Read the model definition and answer for the solid it produces. Units are mm, in the model's axes. A direction names the side the tool comes from. Round coordinates to 2 decimals unless told otherwise and drop trailing zeros. Order: outer loops, then holes, each group sorted by start corner. A loop starts at its lowest first (then second) coordinate and runs counter-clockwise, first axis right, second up. Notation, with made-up numbers: (33.25, 37.25) - (50.25, 37.25) arc R27 cw to (50.25, 75.25) - close; hole circle Ø8 at (-16, 22). An arc over 180 degrees is marked (long way). One line per question, with ' | ' between items. Start each with the question number.
1) Straight lines are drawn through the part: line 1 (X direction, y = 0, z = -6); line 2 (X direction, y = 0, z = -1.3); line 3 (Z direction, x = -1.75, y = 4.5). For each, find the intervals that lie inside material, in ascending order. Write a range as from..to.
2) The mould has two halves that part along Y. Classify faces 4 (the cylindrical face through (-4.783, -1.062, -0.76)), 5 (the flat face through (0, 2, -3.2)), 6 (the flat face through (-1, -4, -1.5)): pulls with the +Y half, pulls with the -Y half, needs draft (parallel to the pull), parting line crosses it, or undercut.
3) Flat-ended cylindrical pins translate along their axes: pin 1 (1 mm diameter, centred on x = 2.5, y = -1, fed in from +Z); pin 2 (1.5 mm diameter, centred on x = 2.5, z = -11.5, fed in from +Y); pin 3 (0.9 mm diameter, centred on x = 0, y = 1, fed in from +Z); pin 4 (2 mm diameter, centred on x = 2.5, z = -3, fed in from -Y). Find the tip coordinate at first contact, or state that the pin passes through.
4) The part is cut by section A-A, the plane x = 0. Give the vertices of the cut face in (y, z), plus the area to 3 significant figures.
5) For faces 1 (the cylindrical face through (0.513, 2.956, -1.622)), 2 (the cylindrical face through (2.64, -2.87, -8.6)), 3 (the flat face through (2, -2, -16)), determine the directions among +Z, -Z, +X, -X, +Y, -Y from which every point of the face is accessible in a straight line to the end or side of a thin tool.
6) The part is cut by section B-B, the plane z = -4.5. Give the vertices of the cut face in (x, y), plus the area to 3 significant figures.
Autodesk Inventor part; units mm, degrees
ref_plane "YZ Plane" through (0, 0, 0) normal (1, 0, 0) x (0, 1, 0)
ref_plane "XZ Plane" through (0, 0, 0) normal (0, 1, 0) x (-1, 0, 0)
ref_plane "XY Plane" through (0, 0, 0) normal (0, 0, 1) x (1, 0, 0)
sketch "Sketch1" plane through (0, 0, 0) normal (1, 0, 0) x (0, 1, 0)
  line L0 (0, 0) -> (1.65, 0) construction
  line L1 (1.65, 0) -> (3, 0) construction
  line L2 (4.9, 0) -> (4.9, -1.5)
  line L3 (4.9, -1.5) -> (3.9, -1.5)
  line L4 (3.9, -1.5) -> (3.9, -16)
  line L5 (3.9, -16) -> (1.7, -16)
  line L6 (1.7, -16) -> (1.7, -3)
  line L7 (0, 0) -> (0, -13.7466) construction
  line L8 (3, 0) -> (3, -3)
  line L9 (3, -3) -> (1.7, -3)
  line L10 (3, 0) -> (4.9, 0)
  dimension "d0" = 1.7
  dimension "d1" = 3.9
  dimension "d2" = 1
  dimension "d3" = 1.5
  dimension "d4" = 14.5
  dimension "d6" = 3
  dimension "d7" = 3
revolve "Revolution1" add sketch "Sketch1" angle 360 about axis through (0, 0, 0) along (0, 0, -1)
fillet "Fillet1" radius 0.5 2 edges at (0, -1.7, -16) (0, -3.9, -16)
sketch "Sketch2" plane through (0, 0, -3) normal (0, 0, 1) x (1, 0, 0)
  circle A0 centre (0, 0) radius 3
  line L0 (-1.7, 2.4718) -> (1.7, 2.4718) construction
  line L1 (1.7, 2.4718) -> (1.7, -2.4718)
  line L2 (1.7, -2.4718) -> (-1.7, -2.4718) construction
  line L3 (-1.7, -2.4718) -> (-1.7, 2.4718)
  circle A1 centre (0, 0) radius 1.7
  point P0 (-1.7, 0)
  point P1 (1.7, 0)
extrude "Extrusion1" cut sketch "Sketch2" against normal blind 0.2 contours L1 A1 L3 A0 | A0 L3 A1 L1
properties part number "HD_BearingShaft2"
Values:
1) line 1: x = -3.9..-1.7, 1.7..3.9 | line 2: x = -4.9..-3, 3..4.9 | line 3: z = -1.5..0
2) face 4: parting line crosses it | face 5: undercut | face 6: needs draft
3) pin 1: stops at z = 0 | pin 2: stops at y = 3.49 | pin 3: passes through | pin 4: stops at y = -3.6
4) outline: (-4.9, -1.5) - (-3.9, -1.5) - (-3.9, -15.5) arc R0.5 ccw to (-3.4, -16) - (-2.2, -16) arc R0.5 ccw to (-1.7, -15.5) - (-1.7, -3.2) - (-3, -3.2) - (-3, 0) - (-4.9, 0) - close; (1.7, -15.5) arc R0.5 ccw to (2.2, -16) - (3.4, -16) arc R0.5 ccw to (3.9, -15.5) - (3.9, -1.5) - (4.9, -1.5) - (4.9, 0) - (3, 0) - (3, -3.2) - (1.7, -3.2) - close | area: 64.9 mm^2
5) face 1: +Z | face 2: -Z | face 3: -Z, +X, -X, +Y, -Y
6) outline: circle Ø7.8 at (0, 0); hole circle Ø3.4 at (0, 0) | area: 38.7 mm^2
